```python
from build123d import *

# Parameters (mm, degrees)
BOSS_EXTRUDE1_DEPTH = 35
SKETCH2_R           = 1.275
CUT_EXTRUDE1_DEPTH  = 5
SKETCH5_R           = 1.65
CUT_EXTRUDE2_DEPTH  = 2
SKETCH6_R           = 1.65
CUT_EXTRUDE3_DEPTH  = 4.175


with BuildPart() as part:
    # Sketch1 → Boss-Extrude1 (new body)
    with BuildSketch(Plane.XY):
        Polygon((0, 0), (19.8, 0), (19.8, -1.7), (18, -1.7), (15.9, -2.9), (15.9, -4.9), (27.3, -4.9), (27.3, 3.175), (-27.3, 3.175), (-27.3, 0), (-20.9, 0), (-20.9, -7.5), (-15.9, -7.5), (-15.9, 0), align=None)
    extrude(amount=BOSS_EXTRUDE1_DEPTH)

    # Sketch2 → Cut-Extrude1 (cut)
    with BuildSketch(Plane.ZY.offset(20.9)):
        with Locations((8.75, -3.75)):
            Circle(SKETCH2_R)
        with Locations((26.25, -3.75)):
            Circle(SKETCH2_R)
    extrude(amount=-CUT_EXTRUDE1_DEPTH, mode=Mode.SUBTRACT)

    # Sketch5 → Cut-Extrude2 (cut)
    with BuildSketch(Plane.XZ):
        Polygon((6.35, 28.354551733), (6.35, 31.645448267), (3.5, 33.290896534), (0.65, 31.645448267), (0.65, 28.354551733), (3.5, 26.709103466), align=None)
        with Locations((3.5, 30)):
            Circle(SKETCH5_R, mode=Mode.SUBTRACT)
        Polygon((-0.65, 6.645448267), (-3.5, 8.290896534), (-6.35, 6.645448267), (-6.35, 3.354551733), (-3.5, 1.709103466), (-0.65, 3.354551733), align=None)
        with Locations((-3.5, 5)):
            Circle(SKETCH5_R, mode=Mode.SUBTRACT)
    extrude(amount=-CUT_EXTRUDE2_DEPTH, mode=Mode.SUBTRACT)

    # Sketch6 → Cut-Extrude3 (cut, through all)
    with BuildSketch(Plane.XZ):
        with Locations((3.5, 30)):
            Circle(SKETCH6_R)
        with Locations((-3.5, 5)):
            Circle(SKETCH6_R)
    extrude(amount=-CUT_EXTRUDE3_DEPTH, mode=Mode.SUBTRACT)


solid = part.part
```
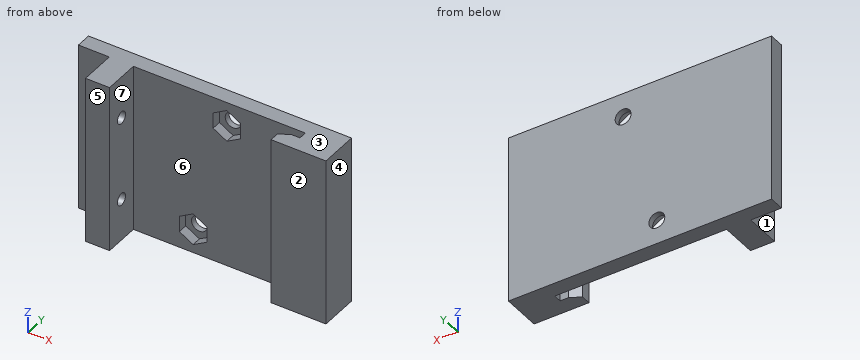
Can you work these out from the model? Positions are in its coordinate system, mm. Face numbers are marked on the shaded views. A direction names the side the tool comes from. Coordinates: 2 decimals unless noted, no trailing zeros. Loops run counter-clockwise (first coordinate to the right, second up) from the corner with the lowest first, then second, coordinate; pieces in that order, holes last. Notation, with made-up numbers: (-1, 87.25) -> (25, 87.25) arc R32 cw to (25, 119.25) -> close; hole circle Ø10 at (-23.5, -17). An arc over 180 degrees is marked (long way). Answer as a JSON object with one key per item and string values.
1) For P1, Ø6, axis at x = 21, z = 13.5, coming from the -Y side; P2, Ø6.5, axis at x = 3.5, z = 29.5, coming from the -Y side; P3, Ø0.6, axis at y = -3.5, z = 16.5, coming from the -X side, each with a flat end and sliding along its axis, tell me the tip position at first contact or that it passes through.
Results:
{"P1": "stops at y = -4.9", "P2": "stops at y = 0", "P3": "stops at x = -20.9"}
2) If I drill on line 1 (X direction, y = 0.25, z = 30.5); line 2 (X direction, y = -4.5, z = 7); line 3 (Z direction, x = 3.5, y = 2.5), over which ranges is the centre line in solid material (lowest first)?
Results:
{"line 1": "x = -27.3 to 0.65, 6.35 to 27.3", "line 2": "x = -20.9 to -15.9, 15.9 to 27.3", "line 3": "z = 0 to 28.35, 31.65 to 35"}
3) For the marked faces 1, 2 and 3, which set-ups out of +Z, -Z, +X, -X, +Y, -Y let a thin tool reach every point of the face, with its end or its side?
Results:
{"face 1": "+Z, -Z, -X, -Y", "face 2": "+Z, -Z, +X, -Y", "face 3": "+Z, +X, -X, +Y, -Y"}
4) Imagine slicing it at A-A (y = -3.75). Please give me the cut outline in (x, z) (3 decimals).
Results:
{"outline": "(-20.9, 0) -> (-15.9, 0) -> (-15.9, 7.475) -> (-20.9, 7.475) -> close; (-20.9, 10.025) -> (-15.9, 10.025) -> (-15.9, 24.975) -> (-20.9, 24.975) -> close; (-20.9, 27.525) -> (-15.9, 27.525) -> (-15.9, 35) -> (-20.9, 35) -> close; (15.9, 0) -> (27.3, 0) -> (27.3, 35) -> (15.9, 35) -> close"}
5) Imagine slicing it at C-C (x = -20). Please give me the cut outline in (y, z) (3 decimals).
Results:
{"outline": "(-7.5, 0) -> (3.175, 0) -> (3.175, 35) -> (-7.5, 35) -> close; hole circle Ø2.55 at (-3.75, 8.75); hole circle Ø2.55 at (-3.75, 26.25)"}
6) Thinking about a two-plate mould opening in X: for the marked faces 4, 5, 6 and 7, which applies, pulls with the +X half, pulls with the -X half, needs draft (parallel to the pull), parting line crosses it, or undercut?
Results:
{"face 4": "pulls with the +X half", "face 5": "needs draft", "face 6": "undercut", "face 7": "undercut"}
7) Imagine slicing it at B-B (z = 19). Please give me the cut outline in (x, y) (3 decimals).
Results:
{"outline": "(-27.3, 0) -> (-20.9, 0) -> (-20.9, -7.5) -> (-15.9, -7.5) -> (-15.9, 0) -> (19.8, 0) -> (19.8, -1.7) -> (18, -1.7) -> (15.9, -2.9) -> (15.9, -4.9) -> (27.3, -4.9) -> (27.3, 3.175) -> (-27.3, 3.175) -> close"}
8) Imagine slicing it at D-D (z = 5). Please give me the cut outline in (x, y) (3 decimals).
Results:
{"outline": "(-27.3, 0) -> (-20.9, 0) -> (-20.9, -7.5) -> (-15.9, -7.5) -> (-15.9, 0) -> (-6.35, 0) -> (-6.35, 2) -> (-5.15, 2) -> (-5.15, 3.175) -> (-27.3, 3.175) -> close; (-1.85, 2) -> (-0.65, 2) -> (-0.65, 0) -> (19.8, 0) -> (19.8, -1.7) -> (18, -1.7) -> (15.9, -2.9) -> (15.9, -4.9) -> (27.3, -4.9) -> (27.3, 3.175) -> (-1.85, 3.175) -> close"}
